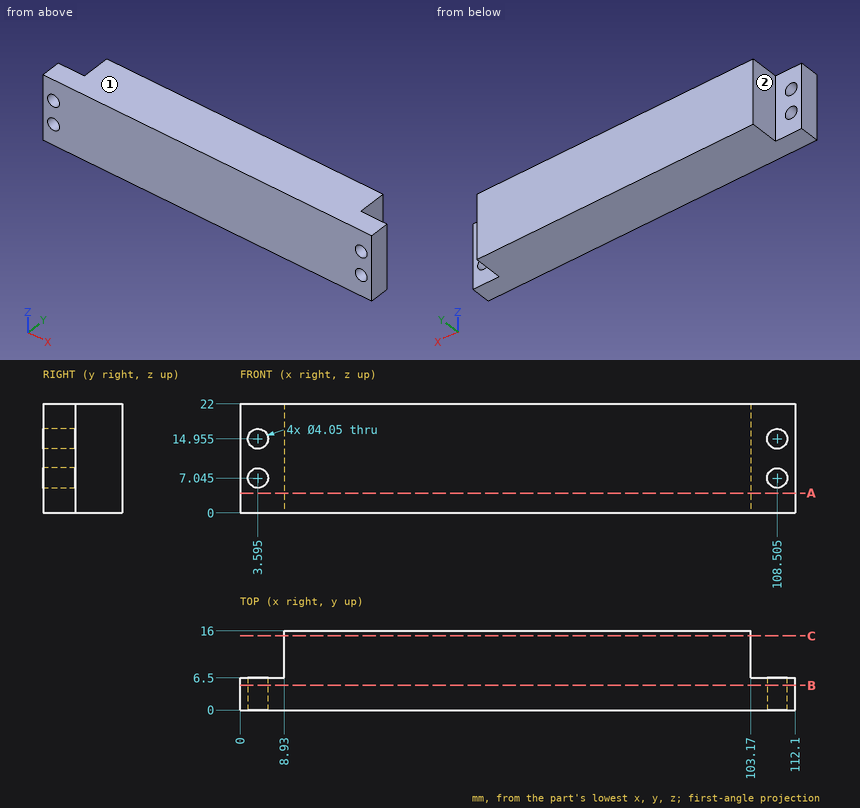
Geometry check sheet. Reference: drawing and pictorial views, mm from the part's lowest x, y, z. A direction names the side the tool comes from. Round coordinates to 2 decimals unless told otherwise and drop trailing zeros. Loops run counter-clockwise (first coordinate to the right, second up) from the corner with the lowest first, then second, coordinate; pieces in that order, holes last. Notation, with made-up numbers: (79, 81.5) - (119, 81.5) arc R13 cw to (119, 102.5) - close; hole circle Ø1 at (-9, -22.75). An arc over 180 degrees is marked (long way). One line per question, with ' | ' between items. Start each with the question number.
1. Tool access check on the marked faces 1 and 2. Record the directions out of +Z, -Z, +X, -X, +Y, -Y that give a thin tool (end or side, any length) a straight path to the whole face; none if there is none.
2. Cross-section at A-A on z = 4. Record the cut outline in (x, y).
3. Scan lines: line 1 (X direction, y = 3.75, z = 14.75); line 2 (X direction, y = 3.25, z = 15.5); line 3 (X direction, y = 14, z = 11). Record each from-to range of solid material in increasing order. Write a range as [from, to].
4. Cross-section at B-B on y = 5. Record the cut outline in (x, z) (3 decimals).
5. Cross-section at C-C on y = 15. Record the cut outline in (x, z), then the cut area to 3 significant figures.
6. Depth check by flat-ended pin: pin 1 (5 mm diameter, centred on y = 12.5, z = 14.5, fed in from -X); pin 2 (7 mm diameter, centred on x = 3, z = 12.5, fed in from +Y); pin 3 (3 mm diameter, centred on y = 9.5, z = 13.5, fed in from +X). Enter the tip coordinate at first touch or a pass-through.
Taken from the geometry:
1) face 1: +Z, +X, -X, +Y, -Y | face 2: +Z, -Z, -X, +Y
2) outline: (0, 0) - (112.1, 0) - (112.1, 6.5) - (103.17, 6.5) - (103.17, 16) - (8.93, 16) - (8.93, 6.5) - (0, 6.5) - close
3) line 1: [0, 1.58], [5.61, 106.49], [110.52, 112.1] | line 2: [0, 1.64], [5.55, 106.55], [110.46, 112.1] | line 3: [8.93, 103.17]
4) outline: (0, 0) - (112.1, 0) - (112.1, 22) - (0, 22) - close; hole circle Ø4.05 at (3.595, 7.045); hole circle Ø4.05 at (3.595, 14.955); hole circle Ø4.05 at (108.505, 7.045); hole circle Ø4.05 at (108.505, 14.955)
5) outline: (8.93, 0) - (103.17, 0) - (103.17, 22) - (8.93, 22) - close | area: 2,070 mm²
6) pin 1: x = 8.93 | pin 2: y = 6.5 | pin 3: x = 103.17
